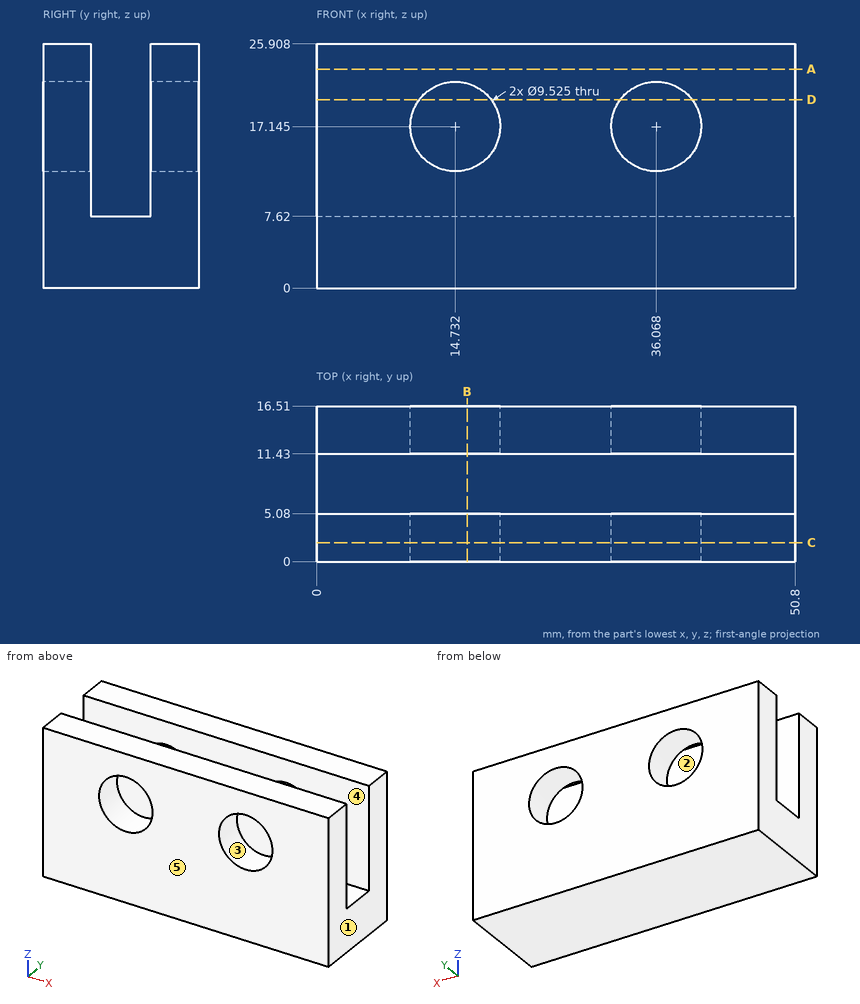
Source: three-view drawing plus pictorial views. Frame: mm from the lowest corner of the part. A direction names the side the tool comes from. Round coordinates to 2 decimals unless told otherwise and drop trailing zeros. Loops run counter-clockwise (first coordinate to the right, second up) from the corner with the lowest first, then second, coordinate; pieces in that order, holes last. Notation, with made-up numbers: (53.5, 42.5) -> (62.5, 42.5) arc R19 ccw to (62.5, 63.5) -> close; hole circle Ø10 at (14, 28). An arc over 180 degrees is marked (long way). Use one line per item in the form item = value.
Item 1: Cut plane A-A on z = 23.25. Output: boundary loops of the cut face in (x, y).
Evaluation:
outline = (0, 0) -> (50.8, 0) -> (50.8, 5.08) -> (0, 5.08) -> close; (0, 11.43) -> (50.8, 11.43) -> (50.8, 16.51) -> (0, 16.51) -> close
Item 2: Cut plane C-C on y = 2. Output: boundary loops of the cut face in (x, z) (1 decimal), then the cut area to 3 significant figures.
Evaluation:
outline = (0, 0) -> (50.8, 0) -> (50.8, 25.9) -> (0, 25.9) -> close; hole circle Ø9.5 at (14.7, 17.1); hole circle Ø9.5 at (36.1, 17.1)
area = 1,170 mm2
Item 3: Cut plane B-B on x = 16. Output: boundary loops of the cut face in (y, z).
Evaluation:
outline = (0, 0) -> (16.51, 0) -> (16.51, 12.55) -> (11.43, 12.55) -> (11.43, 7.62) -> (5.08, 7.62) -> (5.08, 12.55) -> (0, 12.55) -> close; (0, 21.74) -> (5.08, 21.74) -> (5.08, 25.91) -> (0, 25.91) -> close; (11.43, 21.74) -> (16.51, 21.74) -> (16.51, 25.91) -> (11.43, 25.91) -> close
Item 4: Material intervals for probe 1 along Y at (x, z) = (13, 25); probe 2 along X at (y, z) = (12, 16.75); probe 3 along X at (y, z) = (14.75, 15.5), sorted ascending.
Evaluation:
probe_1 = 0 to 5.08, 11.43 to 16.51
probe_2 = 0 to 9.99, 19.48 to 31.32, 40.81 to 50.8
probe_3 = 0 to 10.26, 19.2 to 31.6, 40.54 to 50.8
Item 5: Access query for the marked faces 1 and 2. Directions: +Z, -Z, +X, -X, +Y, -Y. A direction counts if a zero-diameter tool reaches every point of the face in a straight line with its end or side. Return the directions, or none.
Evaluation:
face_1 = +Z, -Z, +X, +Y, -Y
face_2 = +Z, +X, -X
Item 6: Contact query for flat-ended pins moving along their axis: pin 1 Ø5 at (x, y) = (21.5, 7.5) entering from +Z; pin 2 Ø7.5 at (x, z) = (36.068, 17.145) entering from +Y. Output: stop coordinate, or through.
Evaluation:
pin_1 = 25.91
pin_2 = through
Item 7: Draft query along Y for the marked faces 3, 4 and 5. Return one class per face: released by +Y, released by -Y, zero draft, split by the parting line, or undercut.
Evaluation:
face_3 = zero draft
face_4 = undercut
face_5 = released by -Y
Item 8: Cut plane D-D on z = 20. Output: boundary loops of the cut face in (x, y).
Evaluation:
outline = (0, 0) -> (10.92, 0) -> (10.92, 5.08) -> (0, 5.08) -> close; (0, 11.43) -> (10.92, 11.43) -> (10.92, 16.51) -> (0, 16.51) -> close; (18.54, 0) -> (32.26, 0) -> (32.26, 5.08) -> (18.54, 5.08) -> close; (18.54, 11.43) -> (32.26, 11.43) -> (32.26, 16.51) -> (18.54, 16.51) -> close; (39.88, 0) -> (50.8, 0) -> (50.8, 5.08) -> (39.88, 5.08) -> close; (39.88, 11.43) -> (50.8, 11.43) -> (50.8, 16.51) -> (39.88, 16.51) -> close
